```python
from build123d import *

# Parameters (mm, degrees)
F0_R     = 2.3876
F0_W     = 11.9644477963
F0_H     = 25.4
F0_W_2   = 2.794
F0_H_2   = 12.7
F0_H_3   = 18.8976
F1_DEPTH = 3.175
F3_W     = 2.54
F3_H     = 25.4
F4_DEPTH = 2.54
F6_W     = 2.54
F6_H     = 25.4
F7_DEPTH = 2.54


with BuildPart() as f1:
    # F0 (on Front) → F1 (new body, symmetric)
    with BuildSketch(Plane.XZ):
        with BuildLine():
            Line((-9.4017383467, 23.2221963037), (-31.0533456504, 0))
            ThreePointArc((-31.0533456504, 0), (1.5738401562, -75.0292582617), (34.2010259628, 0))
            Line((34.2010259628, 0), (12.5494186591, 23.2221963037))
            Line((12.5494186591, 23.2221963037), (12.5494186591, 43.8596963037))
            Line((12.5494186591, 43.8596963037), (-9.4017383467, 43.8596963037))
            Line((-9.4017383467, 43.8596963037), (-9.4017383467, 23.2221963037))
        make_face()
        with Locations((0, -54.2525947094)):
            Circle(F0_R, mode=Mode.SUBTRACT)
        with Locations((0, -25.0313151628)):
            Rectangle(F0_W, F0_H, mode=Mode.SUBTRACT)
        with Locations((19.9750838982, -56.7813151628)):
            Rectangle(F0_W_2, F0_H_2, mode=Mode.SUBTRACT)
        with Locations((19.9750838982, -28.2825151628)):
            Rectangle(F0_W_2, F0_H_3, mode=Mode.SUBTRACT)
        Polygon((-29.1955699461, -1.7321285843), (-7.5439626424, 21.4900677194), (-5.6861869381, 19.7579391351), (-27.3377942419, -3.4642571686), align=None, mode=Mode.SUBTRACT)
        with Locations((0, 10.739565827)):
            Circle(F0_R, mode=Mode.SUBTRACT)
        Polygon((8.8338672505, 19.7579391351), (10.6916429548, 21.4900677194), (32.3432502585, -1.7321285843), (30.4854745542, -3.4642571686), align=None, mode=Mode.SUBTRACT)
    extrude(amount=F1_DEPTH, both=True)

    # F3 (on offset) → F4 (cut)
    with BuildSketch(Plane(origin=(-16.6122141895, 0, 15.4886787354), x_dir=(0, -1, 0), z_dir=(-0.7314077576, 0, 0.6819403875))):
        with Locations((0, -4.733831039)):
            Rectangle(F3_W, F3_H)
    extrude(amount=-F4_DEPTH, mode=Mode.SUBTRACT)

    # F6 (on offset) → F7 (cut)
    with BuildSketch(Plane(origin=(18.2960887755, 0, 17.0586676721), x_dir=(0, 1, 0), z_dir=(0.7314077576, 0, 0.6819403875))):
        with Locations((0, -6.8803708986)):
            Rectangle(F6_W, F6_H)
    extrude(amount=-F7_DEPTH, mode=Mode.SUBTRACT)


solid = f1.part
```
For this review, take the finished solid that the model builds, in its own axes (mm). A direction names the side the tool comes from. Round coordinates to 2 decimals unless told otherwise and drop trailing zeros. Write each loop counter-clockwise with the first axis right and the second up, starting at its lowest first coordinate (ties: lowest second). Pieces come first, ordered by that corner, then holes. Notation, with made-up numbers: (8, -38) - (17, -38) arc R25 ccw to (17, -19) - close; hole circle Ø9 at (-14, 80.5). An arc over 180 degrees is marked (long way). Use CSV: the item, a comma, the result in double quotes.
1) Add section A-A on z = -32. Write out the cut boundary in (x, y) (3 decimals), and give its area (3 significant figures).
Conclusion:
outline,"(-43.007, -3.175) - (-5.982, -3.175) - (-5.982, 3.175) - (-43.007, 3.175) - close; (5.982, -3.175) - (18.578, -3.175) - (18.578, 3.175) - (5.982, 3.175) - close; (21.372, -3.175) - (46.155, -3.175) - (46.155, 3.175) - (21.372, 3.175) - close"
area,"472 mm^2"
2) For faces 1 (the flat face through (12.549, 0, 33)), 2 (the flat face through (-9.402, 0, 34)), 3 (the flat face through (21.37, -1.46, 10.04)), list the 3-axis set-ups (+Z, -Z, +X, -X, +Y, -Y) from which the entire face can be reached by the end or side of a thin tool; tool diameter is ignored.
Conclusion:
face 1,"+Z, +X, +Y, -Y"
face 2,"+Z, -X, +Y, -Y"
face 3,"+Y, -Y"
3) The part is to be moulded in two halves that separate along Z. For faces 4 (the flat face through (-9, -3.175, -28)), 5 (the cylindrical face through (0, 0, -75)), 6 (the flat face through (-16.36, -0.04, 8.31)), say which applies: pulls with the +Z half, pulls with the -Z half, needs draft (parallel to the pull), parting line crosses it, or undercut.
Conclusion:
face 4,"needs draft"
face 5,"parting line crosses it"
face 6,"undercut"
4) Add section C-C on z = -61. Write out the cut boundary in (x, y) (3 decimals), and give its area (3 significant figures).
Conclusion:
outline,"(-30.904, -3.175) - (18.578, -3.175) - (18.578, 3.175) - (-30.904, 3.175) - close; (21.372, -3.175) - (34.052, -3.175) - (34.052, 3.175) - (21.372, 3.175) - close"
area,"395 mm^2"
5) Add section B-B on x = 0. Write out the cut boundary in (y, z) (3 decimals), and give its area (3 significant figures).
Conclusion:
outline,"(-3.175, -75.001) - (3.175, -75.001) - (3.175, -56.64) - (-3.175, -56.64) - close; (-3.175, -51.865) - (3.175, -51.865) - (3.175, -37.731) - (-3.175, -37.731) - close; (-3.175, -12.331) - (3.175, -12.331) - (3.175, 8.352) - (-3.175, 8.352) - close; (-3.175, 13.127) - (3.175, 13.127) - (3.175, 43.86) - (-3.175, 43.86) - close"
area,"533 mm^2"
6) Clearance check with flat-ended pins moving along their axes: pin 1 Ø3 at (x, y) = (16.5, -2) entering from -Z; pin 2 Ø2 at (x, y) = (19.5, 0) entering from +Z; pin 3 Ø1.9 at (x, y) = (1.5, 1) entering from -Z; pin 4 Ø3 at (x, z) = (0, -54.25) entering from +Y. State where each tip first meets the part, or that it passes through.
Conclusion:
pin 1,"stops at z = -72.96"
pin 2,"stops at z = 9.39"
pin 3,"stops at z = -75.03"
pin 4,"passes through"
7) Add section D-D on z = 25. Write out the cut boundary in (x, y) (3 decimals).
Conclusion:
outline,"(-9.402, -3.175) - (12.549, -3.175) - (12.549, 3.175) - (-9.402, 3.175) - close"
8) Wall thickness on line 1 along X through (y, z) = (2.25, -32.5); line 2 along Z through (x, y) = (0, -0.5) (3 decimals); line 3 along X through (y, z) = (-2, 13.5): over which ranges is each line inside the solid? List them lowest first. Write a range as from..to.
Conclusion:
line 1,"x = -42.99..-5.98, 5.98..18.58, 21.37..46.13"
line 2,"z = -75.001..-56.64, -51.865..-37.731, -12.331..8.352, 13.127..43.86"
line 3,"x = -18.47..-14.99, -11.52..14.67, 18.14..21.61"
